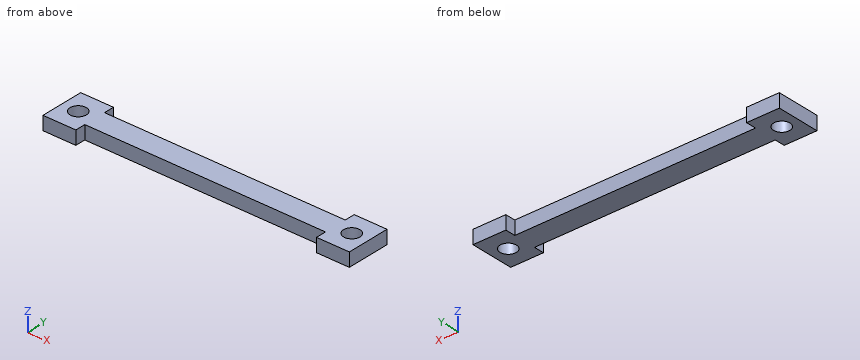
from build123d import *

# Parameters (mm, degrees)
EXTRUDE_1_DEPTH     = 2.5
SKETCH_2_R          = 1.5
CUT_EXTRUDE_1_DEPTH = 2.5


with BuildPart() as part:
    # Эскиз1 → Бобышка-Вытянуть1 (new body)
    with BuildSketch(Plane.XY):
        Polygon((-28, 4), (-22, 4), (-22, 2.1), (22, 2.1), (22, 4), (28, 4), (28, -4), (22, -4), (22, -2.1), (-22, -2.1), (-22, -4), (-28, -4), align=None)
    extrude(amount=EXTRUDE_1_DEPTH)

    # Эскиз2 → Вырез-Вытянуть1 (cut)
    with BuildSketch(Plane.XY.offset(2.5)):
        with Locations((-25, 0)):
            Circle(SKETCH_2_R)
        with Locations(Location((25, 0, 0), (0, 0, 180))):
            Circle(SKETCH_2_R)
    extrude(amount=-CUT_EXTRUDE_1_DEPTH, mode=Mode.SUBTRACT)


solid = part.part
Build history of the part. All positions in model axes, mm. Coordinates: 2 decimals unless noted, no trailing zeros. Write each loop counter-clockwise with the first axis right and the second up, starting at its lowest first coordinate (ties: lowest second). Pieces come first, ordered by that corner, then holes.
(1) Cut at D-D on x = -7.5. List the corners of the cut face in (y, z).
(2) Drill centre lines: line 1 (X direction, y = 2.25, z = 0.9); line 2 (Y direction, x = -25, z = 1.3); line 3 (Y direction, x = 12.5, z = 0.5). Where is each one in solid material? Low to high.
(3) Cut at C-C on z = 0.5. List the corners of the cut face in (x, y), and give its area (3 significant figures).
(4) Pin check, flat tip, straight feed: pin 1 Ø1.8 at (x, y) = (-25, 0) entering from -Z. Stop position of the tip, or through.
(5) Cut at B-B on x = 25. List the corners of the cut face in (y, z), and give its area (3 significant figures).
(6) Cut at A-A on y = 0. List the corners of the cut face in (x, z).
Working result:
1. outline: (-2.1, 0) - (2.1, 0) - (2.1, 2.5) - (-2.1, 2.5) - close
2. line 1: x = -28 to -22, 22 to 28
2. line 2: y = -4 to -1.5, 1.5 to 4
2. line 3: y = -2.1 to 2.1
3. outline: (-28, -4) - (-22, -4) - (-22, -2.1) - (22, -2.1) - (22, -4) - (28, -4) - (28, 4) - (22, 4) - (22, 2.1) - (-22, 2.1) - (-22, 4) - (-28, 4) - close; hole circle Ø3 at (-25, 0); hole circle Ø3 at (25, 0)
3. area: 267 mm2
4. pin 1: passes through
5. outline: (-4, 0) - (-1.5, 0) - (-1.5, 2.5) - (-4, 2.5) - close; (1.5, 0) - (4, 0) - (4, 2.5) - (1.5, 2.5) - close
5. area: 12.5 mm2
6. outline: (-28, 0) - (-26.5, 0) - (-26.5, 2.5) - (-28, 2.5) - close; (-23.5, 0) - (23.5, 0) - (23.5, 2.5) - (-23.5, 2.5) - close; (26.5, 0) - (28, 0) - (28, 2.5) - (26.5, 2.5) - close
